Design review of the part built by this model. Coordinates are the model's own, in mm. A direction names the side the tool comes from. Give positions to 0.01 mm unless a question says otherwise; leave off trailing zeros. Loops run counter-clockwise (first coordinate to the right, second up) from the corner with the lowest first, then second, coordinate; pieces in that order, holes last. Notation, with made-up numbers: (85, 74.25) - (105, 74.25) arc R34 ccw to (105, 113.25) - close; hole circle Ø2 at (11, 47). An arc over 180 degrees is marked (long way). Write each question's results on one line, items separated by ' | '.
Autodesk Inventor part; units mm, degrees
ref_plane "YZ Plane" through (0, 0, 0) normal (1, 0, 0) x (0, 1, 0)
ref_plane "XZ Plane" through (0, 0, 0) normal (0, 1, 0) x (-1, 0, 0)
ref_plane "XY Plane" through (0, 0, 0) normal (0, 0, 1) x (1, 0, 0)
sketch "Sketch1" plane through (0, 0, 0) normal (0, 1, 0) x (-1, 0, 0)
  line L0 (-266.0977, 629.1478) -> (143.9023, 629.1478)
  line L1 (143.9023, 629.1478) -> (143.9023, -80.8522)
  line L2 (143.9023, -80.8522) -> (-266.0977, -80.8522)
  line L3 (-266.0977, -80.8522) -> (-266.0977, 629.1478)
  circle A0 centre (-61.0977, 579.1478) radius 25
  circle A1 centre (-61.0977, -30.8522) radius 25
  point P0 (0, 0)
  dimension "d0" = 710
  dimension "d1" = 410
  dimension "d4" = 50
  dimension "d5" = 50
extrude "Extrusion1" add sketch "Sketch1" along normal blind 3
sketch "Sketch2" plane through (266.0977, 0, 629.1478) normal (1, 0, 0) x (0, 0, -1)
  line L0 (710, 3) -> (0, 3)
  line L1 (710, 3) -> (0, 3)
  line L2 (0, 3) -> (0, 0)
  line L3 (0, 0) -> (710, 0)
  line L4 (710, 0) -> (710, 3)
  line L5 (355, 0) -> (525, 0)
  line L6 (710, 0) -> (0, 0)
  line L7 (355, 3) -> (185, 3)
  line L8 (185, 3) -> (525, 3)
  line L9 (525, 3) -> (525, 0)
  line L10 (525, 0) -> (185, 0)
  line L11 (185, 0) -> (185, 3)
  point P0 (629.1478, 0)
  dimension "d8" = 170
  dimension "d9" = 170
extrude "Extrusion2" add sketch "Sketch2" along normal blind 2000 contours L9 L3 L11 L0
sketch "Sketch3" plane through (0, 3, 0) normal (0, 1, 0) x (1, 0, 0)
  line L0 (2266.0977, -104.1478) -> (2266.0977, -444.1478)
  line L1 (266.0977, -104.1478) -> (2266.0977, -104.1478)
  line L2 (2266.0977, -444.1478) -> (2236.0977, -444.1478)
  line L3 (2236.0977, -444.1478) -> (2236.0977, -104.1478)
  line L4 (2236.0977, -104.1478) -> (2266.0977, -104.1478)
  line L5 (2266.0977, -104.1478) -> (2266.0977, -444.1478)
  point P0 (0, 0)
  dimension "d12" = 340
  dimension "d13" = 30
extrude "Extrusion3" add sketch "Sketch3" along normal blind 200
sketch "Sketch4" plane through (266.0977, 0, 444.1478) normal (0, 0, 1) x (1, 0, 0)
  line L0 (1970, 3) -> (1970, 203)
  line L1 (1970, 203) -> (1970, 2.607)
  line L2 (0, 0) -> (2000, 0)
  line L3 (1970, 203) -> (1758.8495, 2.607)
  line L4 (1758.8495, 2.607) -> (1970, 2.607)
  line L5 (1970, 203) -> (1970, 2.607)
  point P0 (-266.0977, 0)
extrude "Extrusion4" add sketch "Sketch4" against normal blind 30
sketch "Sketch5" plane through (0, 3, 0) normal (0, 1, 0) x (1, 0, 0)
  line L0 (266.0977, 80.8522) -> (-143.9023, 80.8522)
  line L1 (-143.9023, 80.8522) -> (2266.0977, 80.8522)
  line L2 (-143.9023, 80.8522) -> (-143.9023, -629.1478)
  line L3 (-143.9023, 80.8522) -> (-143.9023, -629.1478)
  point P0 (0, 0)
  dimension "d18" = 2410
  dimension "d19" = 710
sketch "Sketch6" plane through (0, 0, 0) normal (0, -1, 0) x (1, 0, 0)
  line L0 (266.0977, 104.1478) -> (2266.0977, 104.1478)
  line L1 (2266.0977, 444.1478) -> (2266.0977, 104.1478)
  line L2 (2266.0977, 104.1478) -> (2266.0977, 444.1478)
  line L3 (2266.0977, 444.1478) -> (266.0977, 444.1478)
  line L4 (-143.9023, 629.1478) -> (266.0977, 629.1478)
  line L5 (266.0977, 444.1478) -> (266.0977, 629.1478)
  line L6 (266.0977, 629.1478) -> (-143.9023, 629.1478)
  line L7 (-143.9023, -80.8522) -> (-143.9023, 629.1478)
  line L8 (-143.9023, 629.1478) -> (-143.9023, -80.8522)
  line L9 (-143.9023, -80.8522) -> (266.0977, -80.8522)
  line L10 (266.0977, 104.1478) -> (266.0977, -80.8522)
  line L11 (266.0977, -80.8522) -> (266.0977, 104.1478)
  line L12 (266.0977, 104.1478) -> (2266.0977, 104.1478)
  circle A0 centre (61.0977, -30.8522) radius 25
  circle A1 centre (61.0977, -30.8522) radius 25
  circle A2 centre (61.0977, 579.1478) radius 25
  circle A3 centre (61.0977, 579.1478) radius 25
  point P0 (0, 0)
extrude "Extrusion5" add sketch "Sketch6" along normal blind 25
sketch "Sketch7" plane through (2236.0977, 3, 104.1478) normal (0, 0, -1) x (-1, 0, 0)
  line L0 (0, 0) -> (0, 200)
  line L1 (1970, -28) -> (-30, -28)
  line L2 (0, 200) -> (-30, 200)
  line L3 (-30, 200) -> (-30, -28)
  line L4 (-30, -28) -> (0, -28)
  line L5 (0, -28) -> (0, 200)
  point P0 (2236.0977, -3)
  point P1 (0, -28)
extrude "Extrusion6" add sketch "Sketch7" along normal blind 200
sketch "Sketch8" plane through (266.0977, 3, 444.1478) normal (0, 0, 1) x (1, 0, 0)
  line L0 (2000, -28) -> (2000, 200)
  line L1 (1970, 200) -> (2000, 200)
  line L2 (2000, -28) -> (1970, -28)
  line L3 (1970, -28) -> (1970, 200)
  line L4 (1970, 200) -> (2000, 200)
  line L5 (2000, 200) -> (2000, -28)
  point P0 (-266.0977, -3)
extrude "Extrusion7" add sketch "Sketch8" along normal blind 200
sketch "Sketch9" plane through (2236.0977, 3, 104.1478) normal (0, 0, -1) x (-1, 0, 0)
  line L0 (0, 200) -> (0, -28)
  line L1 (0, 0) -> (0, 200)
  line L2 (1970, 0) -> (210.7363, 0)
  line L3 (0, 200) -> (210.7363, 0)
  line L4 (210.7363, 0) -> (0, 0)
  point P0 (2236.0977, -3)
extrude "Extrusion8" add sketch "Sketch9" against normal blind 30
properties part number "soporte"
(1) Wall thickness on line 1 along Y through (x, z) = (2, 290); line 2 along X through (y, z) = (140.5, -39.5); line 3 along Z through (x, y) = (1748, -11): over which ranges is each line inside the solid? List them lowest first. Write a range as from..to.
Answers below:
line 1: -25..3 | line 2: 2236.1..2266.1 | line 3: 104.15..444.15
(2) Draft analysis for pull direction Z (two halves, no side actions). For faces 1 (the flat face through (1548, -3, 444.148)), 2 (the flat face through (2132.205, 104.4, 118.938)), 3 (the flat face through (2176, 60, 414.148)), state which applies: pulls with the +Z half, pulls with the -Z half, needs draft (parallel to the pull), parting line crosses it, or undercut.
Answers below:
face 1: pulls with the +Z half | face 2: needs draft | face 3: undercut
(3) Tool access review of faces 4 (the flat face through (2132.205, 104.4, 429.358)), 5 (the flat face through (2236.098, 102, 276)), 6 (the flat face through (1548, -3, 104.148)): name each direction out of +Z, -Z, +X, -X, +Y, -Y from which nothing blocks a thin tool from reaching the whole face with its end or side.
Answers below:
face 4: +Z, -Z, -X, +Y | face 5: -X, +Y | face 6: -Z, +Y, -Y
(4) Insertion check: P1, Ø10, axis at x = 1305.5, z = 367, coming from the +Y side; P2, Ø8.5, axis at x = 158.5, y = -15.5, coming from the -Z side; P3, Ø14, axis at x = 64.5, y = -10.5, coming from the +Z side. Each pin has a flat end and moves straight along its axis. Give the tip position at first contact, or say it passes through.
Answers below:
P1: y = 3 | P2: z = -80.85 | P3: z = 629.15
(5) Take a section at A-A on z = 478. Give the boundary of the cut face in (x, y).
Answers below:
outline: (-143.9, -25) - (266.1, -25) - (266.1, 3) - (-143.9, 3) - close; (2236.1, -25) - (2266.1, -25) - (2266.1, 203) - (2236.1, 203) - close
(6) Take a section at C-C on z = 197. Give the boundary of the cut face in (x, y).
Answers below:
outline: (-143.9, -25) - (2266.1, -25) - (2266.1, 203) - (2236.1, 203) - (2236.1, 3) - (-143.9, 3) - close
(7) Take a section at B-B on y = 165. Give the boundary of the cut face in (x, z), plus the area to 3 significant figures.
Answers below:
outline: (2196.06, 104.15) - (2236.1, 104.15) - (2236.1, -95.85) - (2266.1, -95.85) - (2266.1, 644.15) - (2236.1, 644.15) - (2236.1, 444.15) - (2196.06, 444.15) - (2196.06, 414.15) - (2236.1, 414.15) - (2236.1, 134.15) - (2196.06, 134.15) - close | area: 24,600 mm2
(8) Take a section at D-D on x = 65.5. Give the boundary of the cut face in (y, z).
Answers below:
outline: (-25, -80.85) - (3, -80.85) - (3, -55.46) - (-25, -55.46) - close; (-25, -6.24) - (3, -6.24) - (3, 554.54) - (-25, 554.54) - close; (-25, 603.76) - (3, 603.76) - (3, 629.15) - (-25, 629.15) - close
